Here's how the part is built. I have some questions about the finished solid (model axes, mm). A direction names the side the tool comes from. Give positions to 0.01 mm unless a question says otherwise; leave off trailing zeros. Loops run counter-clockwise (first coordinate to the right, second up) from the corner with the lowest first, then second, coordinate; pieces in that order, holes last. Notation, with made-up numbers: M 71.25,53 L 120.25,53 A22 cw 120.25,62 Z; hole C 15.5,25.5 d7. An arc over 180 degrees is marked long. Answer as CSV lines item,"result". Start each with the question number.
Item 1: If I drill on line 1 along X through (y, z) = (1, 30); line 2 along Y through (x, z) = (3, 24); line 3 along Z through (x, y) = (2.25, -4.5), over which ranges is the centre line in solid material (lowest first)? Write a range as from..to.
Item 2: Will these pins go through, and if not, where does the flat tip stop? P1, Ø3.5, axis at x = -2.5, z = 4.5, coming from the -Y side; P2, Ø1, axis at x = -2, y = -4, coming from the -Z side.
Item 3: I want a section at D-D on z = -30. List the corners of the cut face in (x, y) for me.
Item 4: I want a section at C-C on x = 2. List the corners of the cut face in (y, z) for me.
Item 5: I want a section at A-A on z = 30. List the corners of the cut face in (x, y) for me.
Item 6: I want a section at B-B on y = 3. List the corners of the cut face in (x, z) for me.
Item 7: If we mould it in two halves opening along X, with no side actions, what happens to faces 1 (the cylindrical face through (-4.5, 1.97, -36.07)), 2 (the cylindrical face through (1.819, 1.972, 25.612)), 3 (the cylindrical face through (4.57, 1.97, -36))? For each: released by +X, released by -X, zero draft, split by the parting line, or undercut.
Item 8: For faces 4 (the cylindrical face through (-1.819, -2.712, -25.612)), 5 (the cylindrical face through (-4.57, 1.97, 36)), which set-ups out of +Z, -Z, +X, -X, +Y, -Y let a thin tool reach every point of the face, with its end or its side?
from build123d import *

# Parameters (mm, degrees)
BOSS_EXTRUDE1_DEPTH = 4
SKETCH2_4_R         = 4.75
BOSS_EXTRUDE2_DEPTH = 5.5
SKETCH2_5_R         = 4.75
CUT_EXTRUDE1_DEPTH  = 4


with BuildPart() as part:
    # Sketch2 → Boss-Extrude1 (new body)
    with BuildSketch(Plane(origin=(0, 0, 0), x_dir=(1, 0, 0), z_dir=(0, 1, 0))):
        with BuildLine():
            Line((-1, -37.5), (1, -37.5))
            ThreePointArc((1, -37.5), (4.535533906, -36.035533906), (6, -32.5))
            Line((6, -32.5), (6, 32.5))
            ThreePointArc((6, 32.5), (4.535533906, 36.035533906), (1, 37.5))
            Line((1, 37.5), (-1, 37.5))
            ThreePointArc((-1, 37.5), (-4.535533906, 36.035533906), (-6, 32.5))
            Line((-6, 32.5), (-6, -32.5))
            ThreePointArc((-6, -32.5), (-4.535533906, -36.035533906), (-1, -37.5))
        make_face()
    extrude(amount=BOSS_EXTRUDE1_DEPTH)

    # Sketch2<4> → Boss-Extrude2 (add)
    with BuildSketch(Plane(origin=(0, 0, 0), x_dir=(1, 0, 0), z_dir=(0, 1, 0))):
        with Locations(Location((0, 30, 0), (0, 0, 270))):
            Circle(SKETCH2_4_R)
    extrude(amount=-BOSS_EXTRUDE2_DEPTH)

    # Sketch2<5> → Cut-Extrude1 (cut)
    with BuildSketch(Plane(origin=(0, 0, 0), x_dir=(1, 0, 0), z_dir=(0, 1, 0))):
        with Locations(Location((0, -30, 0), (0, 0, 90))):
            Circle(SKETCH2_5_R)
    extrude(amount=CUT_EXTRUDE1_DEPTH, mode=Mode.SUBTRACT)


solid = part.part
Result:
1,line 1,"-6..-4.75, 4.75..6"
1,line 2,"0..4"
1,line 3,"-34.18..-25.82"
2,P1,"y = 0"
2,P2,"z = -34.51"
3,outline,"M -6,0 L -4.75,0 L -4.75,-5.5 L 4.75,-5.5 L 4.75,0 L 6,0 L 6,4 L -6,4 Z"
4,outline,"M -5.5,-34.31 L 0,-34.31 L 0,-37.4 L 4,-37.4 L 4,25.69 L 0,25.69 L 0,-25.69 L -5.5,-25.69 Z; M 0,34.31 L 4,34.31 L 4,37.4 L 0,37.4 Z"
5,outline,"M -6,0 L -4.75,0 L -4.75,4 L -6,4 Z; M 4.75,0 L 6,0 L 6,4 L 4.75,4 Z"
6,outline,"M -6,-32.5 A5 ccw -1,-37.5 L 1,-37.5 A5 ccw 6,-32.5 L 6,32.5 A5 ccw 1,37.5 L -1,37.5 A5 ccw -6,32.5 Z; hole C 0,30 d9.5"
7,face 1,"released by -X"
7,face 2,"undercut"
7,face 3,"released by +X"
8,face 4,"-Y"
8,face 5,"+Z, -X, +Y, -Y"
